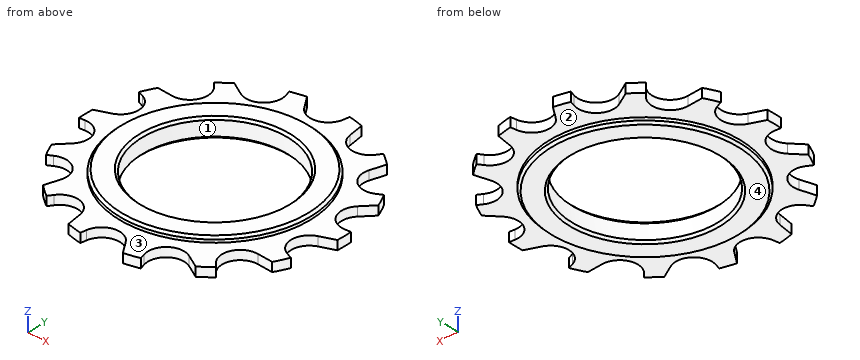
```python
from build123d import *

# Parameters (mm, degrees)
ESQUISSE1_R                  = 28.5
EXTRUSION1_DEPTH             = 1
ENL_V_MAT_EXTRU_1_DEPTH      = 2
R_P_TITION_CIRCULAIRE1_COUNT = 14
ESQUISSE3_R                  = 21
EXTRUSION2_DEPTH             = 2.125
ESQUISSE4_R                  = 16
ENL_V_MAT_EXTRU_2_DEPTH      = 3.125
ENL_V_MAT_EXTRU_2_DEPTH_BACK = 3.125
CHANFREIN1_SIZE              = 0.5


with BuildPart() as part:
    # Esquisse1 → Extrusion1 (new body, symmetric)
    with BuildSketch(Plane.XY):
        Circle(ESQUISSE1_R)
    extrude(amount=EXTRUSION1_DEPTH, both=True)

    # Esquisse2 → Enlèv. mat.-Extru.1 (cut, symmetric)
    with BuildSketch(Plane.XY):
        with BuildLine():
            Line((-5.2427476, 28.013632353), (-3.276608177, 25.205694255))
            ThreePointArc((-3.276608177, 25.205694255), (0.921435362, 23.607576992), (3.957459741, 26.918181818))
            Line((3.957459741, 26.918181818), (4.145454545, 28.196900656))
            ThreePointArc((4.145454545, 28.196900656), (-0.556246195, 28.49457124), (-5.2427476, 28.013632353))
        make_face()
    enl_v_mat_extru_1 = extrude(amount=ENL_V_MAT_EXTRU_1_DEPTH, both=True, mode=Mode.SUBTRACT)

    # Répétition circulaire1: Enlèv. mat.-Extru.1 ×14 about axis
    r_p_tition_circulaire1_axis = Axis((0, 0, 0), (0, 0, 1))
    for i in range(1, R_P_TITION_CIRCULAIRE1_COUNT):
        add(enl_v_mat_extru_1.rotate(r_p_tition_circulaire1_axis, i * 360 / R_P_TITION_CIRCULAIRE1_COUNT), mode=Mode.SUBTRACT)

    # Esquisse3 → Extrusion2 (add, symmetric)
    with BuildSketch(Plane.XY):
        Circle(ESQUISSE3_R)
    extrude(amount=EXTRUSION2_DEPTH, both=True)

    # Esquisse4 → Enlèv. mat.-Extru.2 (cut, two sides)
    with BuildSketch(Plane.XY) as enl_v_mat_extru_2_sk:
        Circle(ESQUISSE4_R)
    extrude(amount=ENL_V_MAT_EXTRU_2_DEPTH, mode=Mode.SUBTRACT)
    extrude(enl_v_mat_extru_2_sk.sketch, amount=-ENL_V_MAT_EXTRU_2_DEPTH_BACK, mode=Mode.SUBTRACT)

    # Chanfrein1
    chanfrein1_edges = [part.edges().sort_by_distance(p)[0] for p in [
        (-21, 0, -2.125),
        (-21, 0, 2.125),
        (-16, 0, -2.125),
        (-16, 0, 2.125),
    ]]
    chamfer(chanfrein1_edges, length=CHANFREIN1_SIZE)


solid = part.part
```
Here's how the part is built. I have some questions about the finished solid (model axes, mm). Face numbers are marked on the shaded views. A direction names the side the tool comes from. Give positions to 0.01 mm unless a question says otherwise; leave off trailing zeros. Order: outer loops, then holes, each group sorted by start corner. A loop starts at its lowest first (then second) coordinate and runs counter-clockwise, first axis right, second up. Notation, with made-up numbers: (81.25, 10.25) -> (86.25, 10.25) arc R23 cw to (86.25, 37.25) -> close; hole circle Ø11 at (15, 76). An arc over 180 degrees is marked (long way). Use CSV: the item, a comma, the result in double quotes. Start each with the question number.
Item 1: Suppose I cut it at A-A (y = 0). List the corners of the cut face in (x, z) for me (3 decimals).
Item 2: Suppose I cut it at B-B (x = 0). List the corners of the cut face in (y, z) for me (3 decimals).
Item 3: I'm going to push flat-ended pins straight in: P1, Ø1.5, axis at x = 18.5, z = 1.5, coming from the -Y side; P2, Ø2, axis at x = -12, z = -0.5, coming from the +Y side. Where does each tip first touch, or does it pass through?
Item 4: If I drill on probe 1 along Y at (x, z) = (0, 0.65); probe 2 along Y at (x, z) = (26, -0.6); probe 3 along Y at (x, z) = (26.5, -0.6), over which ranges is the centre line in solid material (lowest first)? Write a range as [from, to].
Item 5: Thinking about a two-plate mould opening in Y: for the marked faces 1 and 2, which applies, pulls with the +Y half, pulls with the -Y half, needs draft (parallel to the pull), parting line crosses it, or undercut?
Item 6: On a 3-axis mill with a long thin cutter (end or side, diameter ignored), from which of +Z, -Z, +X, -X, +Y, -Y can I reach the whole of each face in a straight line? I mean the marked faces 3 and 4. Say none if no direction works.
Answer block:
1,outline,"(-28.5, -1) -> (-21, -1) -> (-21, -1.625) -> (-20.5, -2.125) -> (-16.5, -2.125) -> (-16, -1.625) -> (-16, 1.625) -> (-16.5, 2.125) -> (-20.5, 2.125) -> (-21, 1.625) -> (-21, 1) -> (-28.5, 1) -> close; (16, -1.625) -> (16.5, -2.125) -> (20.5, -2.125) -> (21, -1.625) -> (21, -1) -> (28.5, -1) -> (28.5, 1) -> (21, 1) -> (21, 1.625) -> (20.5, 2.125) -> (16.5, 2.125) -> (16, 1.625) -> close"
2,outline,"(-23.5, -1) -> (-21, -1) -> (-21, -1.625) -> (-20.5, -2.125) -> (-16.5, -2.125) -> (-16, -1.625) -> (-16, 1.625) -> (-16.5, 2.125) -> (-20.5, 2.125) -> (-21, 1.625) -> (-21, 1) -> (-23.5, 1) -> close; (16, -1.625) -> (16.5, -2.125) -> (20.5, -2.125) -> (21, -1.625) -> (21, -1) -> (23.5, -1) -> (23.5, 1) -> (21, 1) -> (21, 1.625) -> (20.5, 2.125) -> (16.5, 2.125) -> (16, 1.625) -> close"
3,P1,"stops at y = -22.14"
3,P2,"stops at y = 20.92"
4,probe 1,"y = [-23.5, -16], [16, 23.5]"
4,probe 2,"y = [-11.67, -10.1], [-2.13, 2.2], [11.19, 11.67]"
4,probe 3,"y = [-10.49, -10.29], [-1.93, 2.13]"
5,face 1,"undercut"
5,face 2,"needs draft"
6,face 3,"+Z"
6,face 4,"-Z, +X, -X, +Y, -Y"
